Read the model definition and answer for the solid it produces. Units are mm, in the model's axes. Coordinates: 2 decimals unless noted, no trailing zeros. Loops run counter-clockwise (first coordinate to the right, second up) from the corner with the lowest first, then second, coordinate; pieces in that order, holes last. Notation, with made-up numbers: (50, 1) -> (99, 1) arc R14 cw to (99, 21) -> close; hole circle Ø1 at (32, 85). An arc over 180 degrees is marked (long way). Answer in a Markdown table with one row per item.
```python
from build123d import *

# Parameters (mm, degrees)
F1_DEPTH = 10


with BuildPart() as f1:
    # F0 (on Top) → F1 (new body)
    with BuildSketch(Plane.XY):
        Polygon((-125, -111.86579), (-125, -236.247406), (5.863019, -236.247406), (5.863019, -200.747406), (-95, -200.747406), (-95, -111.86579), align=None)
        Polygon((5.863019, -200.747406), (5.863019, -236.247406), (135, -236.247406), (135, -50.747406), (105, -50.747406), (105, -200.747406), align=None)
        Polygon((-125, 134.752594), (-125, -111.86579), (-95, -111.86579), (-95, 99.252594), (15.707426, 99.252594), (15.707426, 134.752594), align=None)
        Polygon((105, -50.747406), (135, -50.747406), (135, 134.752594), (15.707426, 134.752594), (15.707426, 99.252594), (105, 99.252594), align=None)
    extrude(amount=F1_DEPTH)


solid = f1.part
```
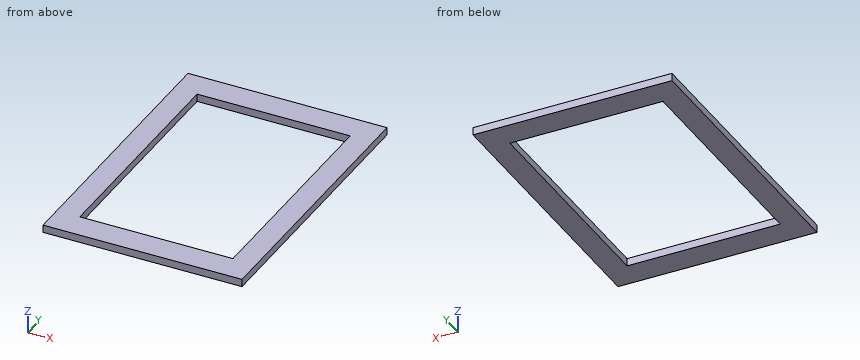
1. A cutting plane is placed at A-A on x = 63. Give the vertices of the cut face in (y, z).
A:
| item | result |
|---|---|
| outline | (-236.25, 0) -> (-200.75, 0) -> (-200.75, 10) -> (-236.25, 10) -> close; (99.25, 0) -> (134.75, 0) -> (134.75, 10) -> (99.25, 10) -> close |
2. A cutting plane is placed at C-C on y = -67. Give the vertices of the cut face in (x, z).
A:
| item | result |
|---|---|
| outline | (-125, 0) -> (-95, 0) -> (-95, 10) -> (-125, 10) -> close; (105, 0) -> (135, 0) -> (135, 10) -> (105, 10) -> close |
3. Find the intervals of material crossed by probe 1 along X at (y, z) = (34.5, 9.5); probe 2 along Y at (x, z) = (-12, 4.75), in increasing order.
A:
| item | result |
|---|---|
| probe 1 | x = -125 to -95, 105 to 135 |
| probe 2 | y = -236.25 to -200.75, 99.25 to 134.75 |
4. A cutting plane is placed at B-B on z = 1.5. Give the vertices of the cut face in (x, y), and give its area (3 significant figures).
A:
| item | result |
|---|---|
| outline | (-125, -236.25) -> (135, -236.25) -> (135, 134.75) -> (-125, 134.75) -> close; hole (-95, -200.75) -> (105, -200.75) -> (105, 99.25) -> (-95, 99.25) -> close |
| area | 36,500 mm2 |
